The model under review builds one solid part; all positions refer to its coordinate system, in mm. A direction names the side the tool comes from. Round coordinates to 2 decimals unless told otherwise and drop trailing zeros. Loops run counter-clockwise (first coordinate to the right, second up) from the corner with the lowest first, then second, coordinate; pieces in that order, holes last. Notation, with made-up numbers: M 89,15 L 123,15 A16 cw 123,30 Z; hole C 48.25,-25 d9. An arc over 180 degrees is marked long. Answer as a JSON object with one key per item and string values. Group by question number.
Item 1: Insertion check: P1, Ø5, axis at y = 8.33, z = 278.76, coming from the -X side; P2, Ø5, axis at y = 8.33, z = 144.15, coming from the +X side; P3, Ø4, axis at x = 8.33, z = 144.15, coming from the +Y side. Each pin has a flat end and moves straight along its axis. Give the tip position at first contact, or say it passes through.
Item 2: To check wall thickness, follow line 1 (X direction, y = 14.25, z = 23). State the ranges of the line that lie inside material, in increasing order.
Item 3: Consider section B-B (x = 13.25). Give the boundary of the cut face in (y, z).
Item 4: Tool access review of faces 1 (the face through (4.4, 0.3, 0)), 2 (the face through (8, 0.794, 175)): name each direction out of +Z, -Z, +X, -X, +Y, -Y from which nothing blocks a thin tool from reaching the whole face with its end or side.
Item 5: Consider section A-A (z = 225.5). Give the boundary of the cut face in (x, y) (3 decimals), and give its area (3 significant figures).
Autodesk Inventor part; units mm, degrees
ref_plane "YZ Plane" through (0, 0, 0) normal (1, 0, 0) x (0, 1, 0)
ref_plane "XZ Plane" through (0, 0, 0) normal (0, 1, 0) x (-1, 0, 0)
ref_plane "XY Plane" through (0, 0, 0) normal (0, 0, 1) x (1, 0, 0)
sketch "Sketch1" plane through (0, 0, 0) normal (0, 0, 1) x (1, 0, 0)
  line L0 (0, 0) -> (0, 15.875)
  line L1 (0, 15.875) -> (0.7937, 15.875)
  line L2 (0.7937, 15.875) -> (0.7938, 0.7937)
  line L3 (0.7938, 0.7937) -> (15.875, 0.7937)
  line L4 (15.875, 0.7937) -> (15.875, 0)
  line L5 (15.875, 0) -> (0, 0)
  dimension "d0" = 15.875
  dimension "d1" = 0.7937
extrude "Extrusion1" add sketch "Sketch1" along normal blind 355.6
sketch "Sketch2" plane through (0.7938, 0.7937, 0) normal (0, 1, 0) x (1, 0, 0)
  line L0 (0, 0) -> (15.0812, 0)
  line L1 (15.0812, -355.6) -> (0, -355.6)
  line L2 (7.5406, 0) -> (7.5406, -355.6) construction
  circle A0 centre (7.5406, -9.525) radius 1.5875
  circle A1 centre (7.5406, -76.835) radius 1.5875
  circle A2 centre (7.5406, -144.145) radius 1.5875
  circle A3 centre (7.5406, -211.455) radius 1.5875
  circle A4 centre (7.5406, -278.765) radius 1.5875
  circle A5 centre (7.5406, -346.075) radius 1.5875
  point P0 (-0.7938, 0)
  dimension "d4" = 9.525
  dimension "d5" = 3.175
  dimension "d6" = 355.6
  dimension "d9" = 67.31
sketch "Sketch3" plane through (0.7938, 0.7937, 0) normal (1, 0, 0) x (0, 0, -1)
  line L0 (0, 15.0812) -> (0, 0)
  line L1 (-355.6, 0) -> (-355.6, 15.0812)
  line L2 (-355.6, 7.5406) -> (0, 7.5406) construction
  circle A0 centre (-9.525, 7.5406) radius 1.5875
  circle A1 centre (-76.835, 7.5406) radius 1.5875
  circle A2 centre (-144.145, 7.5406) radius 1.5875
  circle A3 centre (-211.455, 7.5406) radius 1.5875
  circle A4 centre (-278.765, 7.5406) radius 1.5875
  circle A5 centre (-346.075, 7.5406) radius 1.5875
  point P0 (0, -0.7937)
  dimension "d14" = 3.175
  dimension "d15" = 9.525
  dimension "d16" = 355.6
  dimension "d19" = 67.31
extrude "Extrusion2" cut sketch "Sketch2" against normal through all
extrude "Extrusion3" cut sketch "Sketch3" against normal through all
properties part number "Hopper Bracing Back Bottom P11" material "Aluminum 6061"
Geometry results:
{
 "1": {"P1": "stops at x = 0", "P2": "stops at x = 0.79", "P3": "stops at y = 0.79"},
 "2": {"line 1": "x = 0 to 0.79"},
 "3": {"outline": "M 0,0 L 0.79,0 L 0.79,355.6 L 0,355.6 Z"},
 "4": {"face 1": "-Z, +X, -X, +Y, -Y", "face 2": "+Z, -Z, +X, +Y"},
 "5": {"outline": "M 0,0 L 15.875,0 L 15.875,0.794 L 0.794,0.794 L 0.794,15.875 L 0,15.875 Z", "area": "24.6 mm^2"}
}
